from build123d import *

# Parameters (mm, degrees)
F1_DEPTH = 10


with BuildPart() as f1:
    # F0 (on Top) → F1 (new body)
    with BuildSketch(Plane.XY):
        with BuildLine():
            ThreePointArc((-58.746551, 11.539105), (-8.024476, 87.805772), (42.697599, 11.539105))
            Line((42.697599, 11.539105), (20.749777, -40.807561))
            ThreePointArc((20.749777, -40.807561), (20.83933, -41.748003), (21.671996, -42.194228))
            Line((21.671996, -42.194228), (22.756337, -42.194228))
            ThreePointArc((22.756337, -42.194228), (23.310112, -42.026894), (23.678556, -41.580895))
            Line((23.678556, -41.580895), (45.464258, 10.379105))
            ThreePointArc((45.464258, 10.379105), (-8.024476, 90.805772), (-61.513209, 10.379105))
            Line((-61.513209, 10.379105), (-39.727507, -41.580895))
            ThreePointArc((-39.727507, -41.580895), (-39.359063, -42.026894), (-38.805288, -42.194228))
            Line((-38.805288, -42.194228), (-37.720947, -42.194228))
            ThreePointArc((-37.720947, -42.194228), (-36.888281, -41.748003), (-36.798728, -40.807561))
            Line((-36.798728, -40.807561), (-58.746551, 11.539105))
        make_face()
    extrude(amount=F1_DEPTH)


solid = f1.part
Design review of the part built by this model. Coordinates are the model's own, in mm. A direction names the side the tool comes from. Round coordinates to 2 decimals unless told otherwise and drop trailing zeros. Write each loop counter-clockwise with the first axis right and the second up, starting at its lowest first coordinate (ties: lowest second). Pieces come first, ordered by that corner, then holes. Notation, with made-up numbers: M 16.5,4.25 L 61.5,4.25 A20 cw 61.5,30.25 Z; hole C 77,73.25 d9. An arc over 180 degrees is marked long. One line per item, written item: value. Start each with the question number.
1. To check wall thickness, follow probe 1 along X at (y, z) = (32, 2.5); probe 2 along X at (y, z) = (-10.5, 9.25); probe 3 along Y at (x, z) = (-53, 1.75). State the ranges of each line that lie inside material, in increasing order. Write a range as from..to.
2. For faces 1 (the face through (-47.62, -15, 4.93)), 2 (the face through (13, 84, 0)), list the 3-axis set-ups (+Z, -Z, +X, -X, +Y, -Y) from which the entire face can be reached by the end or side of a thin tool; tool diameter is ignored.
3. Take a section at C-C on z = 5.25. State the section outline as (x, y) points.
4. Clearance check with flat-ended pins moving along their axes: P1, Ø1, axis at y = 20, z = 5, coming from the -X side; P2, Ø3, axis at y = 11.5, z = 3, coming from the -X side; P3, Ø1.5, axis at y = 1, z = 2.5, coming from the +X side. State where each tip first meets the part, or that it passes through.
5. Take a section at B-B on y = 42.5. State the section outline as (x, z) points.
6. Take a section at D-D on x = -33.5. State the section outline as (y, z) points.
7. Draft analysis for pull direction X (two halves, no side actions). For faces 3 (the face through (34.42, -15.96, 4.93)), 4 (the face through (31.877, -14.268, 4.93)), 5 (the face through (-9.539, 87.785, 4.93)), 6 (the face through (-6.427, 90.784, 4.93)), state which applies: pulls with the +X half, pulls with the -X half, needs draft (parallel to the pull), parting line crosses it, or undercut.
8. Take a section at A-A on x = -51. State the section outline as (y, z) points, then the cut area to 3 significant figures.
Computed:
1. probe 1: x = -66.02..-63.02, 46.97..49.97
1. probe 2: x = -52.76..-49.51, 33.46..36.71
1. probe 3: y = -9.93..-2.17, 64.46..69.43
2. face 1: +Z, -Z
2. face 2: -Z, +X, -X, +Y, -Y
3. outline: M -61.51,10.38 L -39.73,-41.58 A1 ccw -38.81,-42.19 L -37.72,-42.19 A1 ccw -36.8,-40.81 L -58.75,11.54 A55 cw long 42.7,11.54 L 20.75,-40.81 A1 ccw 21.67,-42.19 L 22.76,-42.19 A1 ccw 23.68,-41.58 L 45.46,10.38 A58 ccw long Z
4. P1: stops at x = -64.7
4. P2: stops at x = -62.54
4. P3: stops at x = 41.85
5. outline: M -65.21,0 L -62.16,0 L -62.16,10 L -65.21,10 Z; M 46.11,0 L 49.16,0 L 49.16,10 L 46.11,10 Z
6. outline: M 81.55,0 L 84.91,0 L 84.91,10 L 81.55,10 Z
7. face 3: pulls with the +X half
7. face 4: undercut
7. face 5: undercut
7. face 6: parting line crosses it
8. outline: M -14.7,0 L -6.94,0 L -6.94,10 L -14.7,10 Z; M 67.13,0 L 71.76,0 L 71.76,10 L 67.13,10 Z
8. area: 124 mm²
